Verification items for the finished model (mm, model axes). A direction names the side the tool comes from. Round coordinates to 2 decimals unless told otherwise and drop trailing zeros. Write each loop counter-clockwise with the first axis right and the second up, starting at its lowest first coordinate (ties: lowest second). Pieces come first, ordered by that corner, then holes.
from build123d import *

# Parameters (mm, degrees)
BOSS_EXTRUDE1_DEPTH = 5


with BuildPart() as part:
    # Sketch1 → Boss-Extrude1 (new body)
    with BuildSketch(Plane.XY):
        with BuildLine():
            Line((-232.377693895, 91.946298682), (-172.366969932, 243.677851947))
            ThreePointArc((-172.366969932, 243.677851947), (-168.690205127, 248.269779909), (-163.067862176, 250))
            Line((-163.067862176, 250), (-0.1, 250))
            Line((-0.1, 250), (163.075862176, 250))
            ThreePointArc((163.075862176, 250), (168.693678089, 248.272855877), (172.370938455, 243.688028873))
            Line((172.370938455, 243.688028873), (232.476906979, 92.200721814))
            ThreePointArc((232.476906979, 92.200721814), (0.236829395, -249.999962555), (-232.377693895, 91.946298682))
        make_face()
        with BuildLine():
            Line((15.838692049, -47.319613631), (57.786513592, -105.055836805))
            ThreePointArc((57.786513592, -105.055836805), (0, -119.9), (-57.786513592, -105.055836805))
            Line((-57.786513592, -105.055836805), (-15.838692049, -47.319613631))
            ThreePointArc((-15.838692049, -47.319613631), (0, -49.9), (15.838692049, -47.319613631))
        make_face(mode=Mode.SUBTRACT)
        with BuildLine():
            Line((-40.10920188, -29.686056062), (-82.057023423, -87.422279237))
            ThreePointArc((-82.057023423, -87.422279237), (-114.031676304, -37.051137626), (-117.771052914, 22.494201374))
            Line((-117.771052914, 22.494201374), (-49.898051904, 0.440926504))
            ThreePointArc((-49.898051904, 0.440926504), (-47.457720163, -15.419948019), (-40.10920188, -29.686056062))
        make_face(mode=Mode.SUBTRACT)
        with BuildLine():
            Line((40.10920188, -29.686056062), (82.057023423, -87.422279237))
            ThreePointArc((82.057023423, -87.422279237), (114.031676304, -37.051137626), (117.771052914, 22.494201374))
            Line((117.771052914, 22.494201374), (49.898051904, 0.440926504))
            ThreePointArc((49.898051904, 0.440926504), (47.457720163, -15.419948019), (40.10920188, -29.686056062))
        make_face(mode=Mode.SUBTRACT)
        with BuildLine():
            Line((-137.21255284, 60.354994352), (-204.01494883, 82.060408564))
            ThreePointArc((-204.01494883, 82.060408564), (-129.253976979, 177.902837063), (-15, 219.387807318))
            Line((-15, 219.387807318), (-15, 149.147611446))
            ThreePointArc((-15, 149.147611446), (-88.109009319, 121.271647457), (-137.21255284, 60.354994352))
        make_face(mode=Mode.SUBTRACT)
        with BuildLine():
            Line((-146.483062671, 31.823298863), (-213.285458662, 53.528713076))
            ThreePointArc((-213.285458662, 53.528713076), (-209.137327933, -67.952837063), (-141.08817259, -168.671685695))
            Line((-141.08817259, -168.671685695), (-99.802021338, -111.846173546))
            ThreePointArc((-99.802021338, -111.846173546), (-142.563371793, -46.321647457), (-146.483062671, 31.823298863))
        make_face(mode=Mode.SUBTRACT)
        with BuildLine():
            Line((-75.531511507, -129.479731115), (-116.817662759, -186.305243264))
            ThreePointArc((-116.817662759, -186.305243264), (0, -219.9), (116.817662759, -186.305243264))
            Line((116.817662759, -186.305243264), (75.531511507, -129.479731115))
            ThreePointArc((75.531511507, -129.479731115), (0, -149.9), (-75.531511507, -129.479731115))
        make_face(mode=Mode.SUBTRACT)
        with BuildLine():
            Line((99.802021338, -111.846173546), (141.08817259, -168.671685695))
            ThreePointArc((141.08817259, -168.671685695), (209.137327933, -67.952837063), (213.285458662, 53.528713076))
            Line((213.285458662, 53.528713076), (146.483062671, 31.823298863))
            ThreePointArc((146.483062671, 31.823298863), (142.563371793, -46.321647457), (99.802021338, -111.846173546))
        make_face(mode=Mode.SUBTRACT)
        with BuildLine():
            Line((137.21255284, 60.354994352), (204.01494883, 82.060408564))
            ThreePointArc((204.01494883, 82.060408564), (129.253976979, 177.902837063), (15, 219.387807318))
            Line((15, 219.387807318), (15, 149.147611446))
            ThreePointArc((15, 149.147611446), (88.109009319, 121.271647457), (137.21255284, 60.354994352))
        make_face(mode=Mode.SUBTRACT)
        with BuildLine():
            Line((15, 47.592121197), (15, 118.958017805))
            ThreePointArc((15, 118.958017805), (70.47545175, 97.001137626), (108.500543083, 51.025896863))
            Line((108.500543083, 51.025896863), (40.627542073, 28.972621993))
            ThreePointArc((40.627542073, 28.972621993), (29.330484089, 40.369948019), (15, 47.592121197))
        make_face(mode=Mode.SUBTRACT)
        with BuildLine():
            Line((-40.627542073, 28.972621993), (-108.500543083, 51.025896863))
            ThreePointArc((-108.500543083, 51.025896863), (-70.47545175, 97.001137626), (-15, 118.958017805))
            Line((-15, 118.958017805), (-15, 47.592121197))
            ThreePointArc((-15, 47.592121197), (-29.330484089, 40.369948019), (-40.627542073, 28.972621993))
        make_face(mode=Mode.SUBTRACT)
    extrude(amount=BOSS_EXTRUDE1_DEPTH)


solid = part.part
Q1. Release check for a two-part mould opening along Y. For faces 3 (the flat face through (4, 4, 0)), 4 (the flat face through (-202.792, 166.75, 2.465)), 5 (the cylindrical face through (-29.15, 40.5, 2.46)) record: released by +Y, released by -Y, zero draft, split by the parting line, or undercut.
Recorded:
face 3: zero draft
face 4: released by +Y
face 5: undercut
Q2. Depth check by flat-ended pin: P1, Ø2.5, axis at y = 190, z = 1.5, coming from the +X side; P2, Ø3, axis at y = 147, z = 4, coming from the +X side. Enter the tip coordinate at first touch or a pass-through.
Recorded:
P1: stops at x = 194.17
P2: stops at x = 211.33
Q3. Sectioned sample at D-D (y = 175.5). Enter the section's corners in (x, z), plus the area to 3 significant figures.
Recorded:
outline: (-199.33, 0) - (-132.5, 0) - (-132.5, 5) - (-199.33, 5) - close; (-15, 0) - (15, 0) - (15, 5) - (-15, 5) - close; (132.5, 0) - (199.43, 0) - (199.43, 5) - (132.5, 5) - close
area: 819 mm2
Q4. Tool access check on faces 1 (the flat face through (4, 4, 5)), 2 (the cylindrical face through (-130.645, 176.884, 2.465)). Record the directions out of +Z, -Z, +X, -X, +Y, -Y that give a thin tool (end or side, any length) a straight path to the whole face; none if there is none.
Recorded:
face 1: +Z, +X, -X, +Y, -Y
face 2: +Z, -Z
Q5. Sectioned sample at C-C (y = -194.5). Enter the section's corners in (x, z).
Recorded:
outline: (-156.97, 0) - (-102.6, 0) - (-102.6, 5) - (-156.97, 5) - close; (102.6, 0) - (157.17, 0) - (157.17, 5) - (102.6, 5) - close
Q6. Sectioned sample at B-B (x = 0.1). Enter the section's corners in (y, z).
Recorded:
outline: (-250, 0) - (-219.9, 0) - (-219.9, 5) - (-250, 5) - close; (-149.9, 0) - (-119.9, 0) - (-119.9, 5) - (-149.9, 5) - close; (-49.9, 0) - (250, 0) - (250, 5) - (-49.9, 5) - close
Q7. Material ranges on line 1 along Y through (x, z) = (-91, 3.95); line 2 along X through (y, z) = (-58.5, 1.25); line 3 along Y through (x, z) = (-88.5, 0.6), recorded low to high.
Recorded:
line 1: y = -232.81 to -200.19, -150.77 to -78.07, 13.8 to 45.34, 78.07 to 119.12, 200.19 to 250
line 2: x = -242.96 to -211.98, -138.01 to -104.66, -61.04 to -23.96, 23.96 to 61.04, 104.66 to 138.01, 211.98 to 243.16
line 3: y = -233.77 to -201.31, -147.33 to -80.89, 12.98 to 44.53, 80.89 to 120.99, 201.31 to 250
Q8. Sectioned sample at A-A (y = -71). Enter the section's corners in (x, z).
Recorded:
outline: (-239.61, 0) - (-208.12, 0) - (-208.12, 5) - (-239.61, 5) - close; (-132.02, 0) - (-96.62, 0) - (-96.62, 5) - (-132.02, 5) - close; (-70.13, 0) - (-33.04, 0) - (-33.04, 5) - (-70.13, 5) - close; (33.04, 0) - (70.13, 0) - (70.13, 5) - (33.04, 5) - close; (96.62, 0) - (132.02, 0) - (132.02, 5) - (96.62, 5) - close; (208.12, 0) - (239.81, 0) - (239.81, 5) - (208.12, 5) - close
